```python
from build123d import *

# Parameters (mm, degrees)
BOSS_EXTRUDE1_DEPTH = 160


with BuildPart() as part:
    # Sketch4 → Boss-Extrude1 (new body, symmetric)
    with BuildSketch(Plane.XY):
        with BuildLine():
            Line((4.8, -20), (17.2, -20))
            ThreePointArc((17.2, -20), (19.179898987, -19.179898987), (20, -17.2))
            Line((20, -17.2), (20, -4.8))
            ThreePointArc((20, -4.8), (19.765685425, -4.234314575), (19.2, -4))
            Line((19.2, -4), (16.190663761, -4))
            ThreePointArc((16.190663761, -4), (15.624978336, -4.234314575), (15.390663761, -4.8))
            Line((15.390663761, -4.8), (15.390663761, -10.2))
            ThreePointArc((15.390663761, -10.2), (14.896810507, -10.939103626), (14.024978336, -10.765685425))
            Line((14.024978336, -10.765685425), (9.40588745, -6.146594539))
            ThreePointArc((9.40588745, -6.146594539), (8.365378244, -4.589362465), (8, -2.752481989))
            Line((8, -2.752481989), (8, 0))
            Line((8, 0), (3.5, 0))
            ThreePointArc((3.5, 0), (2.474873734, -2.474873734), (0, -3.5))
            Line((0, -3.5), (0, -8))
            Line((0, -8), (2.752481989, -8))
            ThreePointArc((2.752481989, -8), (4.589362465, -8.365378244), (6.146594539, -9.40588745))
            Line((6.146594539, -9.40588745), (10.765685425, -14.024978336))
            ThreePointArc((10.765685425, -14.024978336), (10.939103626, -14.896810507), (10.2, -15.390663761))
            Line((10.2, -15.390663761), (4.8, -15.390663761))
            ThreePointArc((4.8, -15.390663761), (4.234314575, -15.624978336), (4, -16.190663761))
            Line((4, -16.190663761), (4, -19.2))
            ThreePointArc((4, -19.2), (4.234314575, -19.765685425), (4.8, -20))
        make_face()
    extrude(amount=BOSS_EXTRUDE1_DEPTH, both=True)

    # Mirror1: part across plane


with BuildPart() as part_1:
    add(part.part)
    add(part.part.mirror(Plane(origin=(0, 0, 0), x_dir=(0, 0, 1), z_dir=(1, 0, 0))))

    # Mirror2: part across plane


with BuildPart() as part_2:
    add(part_1.part)
    add(part_1.part.mirror(Plane.ZX))


solid = part_2.part
```
Source: CAD feature listing. Evaluate the final solid. Frame: model axes, mm. A direction names the side the tool comes from. Give positions to 0.01 mm unless a question says otherwise; leave off trailing zeros.
1. Access query for faces 1 (the face through (8, 0, 2)), 2 (the face through (20, -11, 2)), 3 (the face through (15.391, -7, 2)), 4 (the face through (-8, 0, 2)), 5 (the face through (0, -8, 2)). Directions: +Z, -Z, +X, -X, +Y, -Y. A direction counts if a zero-diameter tool reaches every point of the face in a straight line with its end or side. Return the directions, or none.
2. Material intervals for line 1 along Y through (x, z) = (7, -59.5); line 2 along Y through (x, z) = (16, -24.5); line 3 along X through (y, z) = (-14, 24), sorted ascending.
3. Pull-direction query (X, two-part tool) for faces 6 (the face through (-20, 11, 2)), 7 (the face through (-11, 20, 2)), 8 (the face through (0, 8, 2)); classes: +X half, -X half, draft (parallel to the pull), parting line (faces both ways), or undercut.
4. First-contact query: pin 1 (3 mm diameter, centred on y = -0.5, z = -30.5, fed in from +X); pin 2 (3.5 mm diameter, centred on x = -17.5, z = 21, fed in from -Y); pin 3 (1.5 mm diameter, centred on x = -3.5, z = -29, fed in from -Y); pin 4 (0.9 mm diameter, centred on y = -18, z = -51, fed in from +X). Flat tips, straight axial feed; report the tip coordinate or a pass-through.
Output values:
1. face 1: +Z, -Z, +X
1. face 2: +Z, -Z, +X, +Y, -Y
1. face 3: +Z, -Z
1. face 4: +Z, -Z, -X
1. face 5: +Z, -Z, -Y
2. line 1: y = -20 to -15.39, -10.26 to 10.26, 15.39 to 20
2. line 2: y = -20 to -4.02, 4.02 to 20
2. line 3: x = -20 to -10.74, 10.74 to 20
3. face 6: -X half
3. face 7: draft
3. face 8: undercut
4. pin 1: stops at x = 8
4. pin 2: stops at y = -20
4. pin 3: stops at y = -19.78
4. pin 4: stops at x = 19.98
